Source: CAD feature listing. Evaluate the final solid. Frame: model axes, mm. A direction names the side the tool comes from. Coordinates: 2 decimals unless noted, no trailing zeros. Order: outer loops, then holes, each group sorted by start corner. A loop starts at its lowest first (then second) coordinate and runs counter-clockwise, first axis right, second up.
Item 1: Mould query, pull axis Y, two halves, no side actions, for faces 1 (the flat face through (12.98, 25.55, -54.55)), 2 (the cylindrical face through (15.63, 30.55, -67.76)), 3 (the flat face through (0, 10, -55)). Classes: released by +Y, released by -Y, zero draft, split by the parting line, or undercut.
Item 2: Section B-B on x = 1. Return the cut outline in (y, z).
Item 3: Section C-C on y = 25.5. Return the cut outline in (x, z).
Item 4: Section A-A on z = -2.62. Return the cut outline in (x, y).
Item 5: Ray query, line 1 (X direction, y = 6, z = -2.62); line 2 (Z direction, x = -5, y = 12); line 3 (X direction, y = 19, z = -33.5). Return the intervals inside material, ascending.
Item 6: Section D-D on z = -25. Return the cut outline in (x, y).
Item 7: Contact query for flat-ended pins moving along their axis: P1, Ø7, axis at y = 31, z = -61.5, coming from the -X side; P2, Ø1, axis at x = -3, z = -59.5, coming from the +Y side; P3, Ø8, axis at x = 0.5, z = -43.5, coming from the +Y side; P4, Ø8, axis at x = 2.5, z = -71, coming from the +Y side. Output: stop coordinate, or through.
Item 8: Reachability of faces 4 (the flat face through (13, 28, -50.07)), 5 (the flat face through (0, 29.5, -68)), 6 (the flat face through (0, 10, -6.622)), 7 (the flat face through (15.5, 12, -23)) from +Z, -Z, +X, -X, +Y, -Y: full face, straight path, thin tool, end or side. Return the list, or none.
from build123d import *

# Parameters (mm, degrees)
SKETCH1_W                  = 32
SKETCH1_H                  = 78.52
BOSS_EXTRUDE1_DEPTH        = 4
M3_CLEARANCE_HOLE1_D       = 3.6
M3_CLEARANCE_HOLE1_DEPTH   = 10
M3_CLEARANCE_HOLE1_TIP     = 1.081549114
BOSS_EXTRUDE2_DEPTH        = 17
BOSS_EXTRUDE3_DEPTH        = 17
SKETCH6_W                  = 32
SKETCH6_H                  = 1.5
SKETCH6_W_2                = 4
SKETCH6_H_2                = 6
BOSS_EXTRUDE4_DEPTH        = 8.5
SKETCH14_W                 = 4
SKETCH14_H                 = 18.45
BOSS_EXTRUDE5_DEPTH        = 6
FILLET1_R                  = 5
CHAMFER1_SIZE              = 3
CHAMFER2_SIZE              = 3
CUT_EXTRUDE1_DEPTH         = 87.102499383
CUT_EXTRUDE1_DEPTH_BACK    = 87.102499383
SKETCH15_W                 = 21
SKETCH15_H                 = 40.897809358
F_5_3_5_3_DIAMETER_HOLE1_D = 5.3
SKETCH19_W                 = 21
SKETCH19_H                 = 12
CUT_EXTRUDE2_DEPTH         = 10
CUT_EXTRUDE3_DEPTH         = 83.839546112
CUT_EXTRUDE3_DEPTH_BACK    = 83.839546112
SKETCH20_W                 = 6
SKETCH20_H                 = 2
CHAMFER3_SIZE              = 8.984147096
CHAMFER3_SIZE_2            = 4


with BuildPart() as part:
    # Sketch1 → Boss-Extrude1 (new body)
    with BuildSketch(Plane(origin=(0, 0, 0), x_dir=(1, 0, 0), z_dir=(0, 1, 0))):
        with Locations((0, 39.26)):
            Rectangle(SKETCH1_W, SKETCH1_H)
    extrude(amount=BOSS_EXTRUDE1_DEPTH)

    # M3 Clearance Hole1
    with Locations(Plane(origin=(0, 4, 0), x_dir=(1, 0, 0), z_dir=(0, 1, 0))):
        with Locations((-10, 73.52), (10, 73.52)):
            Hole(M3_CLEARANCE_HOLE1_D / 2, depth=M3_CLEARANCE_HOLE1_DEPTH)
            with Locations((0, 0, -(M3_CLEARANCE_HOLE1_DEPTH + M3_CLEARANCE_HOLE1_TIP / 2))):  # 118° drill point
                Cone(0, M3_CLEARANCE_HOLE1_D / 2, M3_CLEARANCE_HOLE1_TIP, mode=Mode.SUBTRACT)

    # Sketch5 → Boss-Extrude2 (add)
    with BuildSketch(Plane(origin=(0, 4, 0), x_dir=(1, 0, 0), z_dir=(0, 1, 0))):
        Polygon((16, 68.52), (-16, 68.52), (-16, 47.520000358), (-15.5, 47.520000358), (-10.5, 47.520000358), (10.5, 47.520000358), (15.5, 47.520000358), (16, 47.520000358), align=None)
    extrude(amount=BOSS_EXTRUDE2_DEPTH)

    # Sketch5<4> → Boss-Extrude3 (add)
    with BuildSketch(Plane(origin=(0, 4, 0), x_dir=(1, 0, 0), z_dir=(0, 1, 0))):
        Polygon((-10.5, 47.520000358), (-15.5, 47.520000358), (-15.5, 0), (15.5, 0), (15.5, 47.520000358), (10.5, 47.520000358), (10.5, 6.622191), (-10.5, 6.622191), align=None)
    extrude(amount=BOSS_EXTRUDE3_DEPTH)

    # Sketch6 → Boss-Extrude4 (add)
    with BuildSketch(Plane(origin=(0, 21, 0), x_dir=(1, 0, 0), z_dir=(0, 1, 0))):
        with Locations((0, 67.77)):
            Rectangle(SKETCH6_W, SKETCH6_H)
        with Locations((13.5, 53.07)):
            Rectangle(SKETCH6_W_2, SKETCH6_H_2)
        with Locations((-13.5, 53.07)):
            Rectangle(SKETCH6_W_2, SKETCH6_H_2)
    extrude(amount=BOSS_EXTRUDE4_DEPTH)

    # Sketch14 → Boss-Extrude5 (add)
    with BuildSketch(Plane(origin=(0, 29.5, 0), x_dir=(1, 0, 0), z_dir=(0, 1, 0))):
        with Locations((-13.5, 59.295)):
            Rectangle(SKETCH14_W, SKETCH14_H)
        with Locations((13.5, 59.295)):
            Rectangle(SKETCH14_W, SKETCH14_H)
    extrude(amount=BOSS_EXTRUDE5_DEPTH)

    # Fillet1
    # the kernel refuses this fillet: 5 mm, written as the material it adds along each edge
    with BuildSketch(Plane(origin=(-11.5, 29.5, -68.52), x_dir=(0, 1, 0), z_dir=(0, 0, 1)), Plane(origin=(11.5, 29.5, -68.52), x_dir=(-1, 0, 0), z_dir=(0, 0, 1))) as fillet1_piece_1:
        with BuildLine():
            CenterArc((FILLET1_R, -FILLET1_R), FILLET1_R, 90, 90)
            Line((0, -FILLET1_R), (0, 0))
            Line((0, 0), (FILLET1_R, 0))
        make_face()
    extrude(amount=1.5)
    with BuildSketch(Plane(origin=(-15.5, 29.5, -67.02), x_dir=(-1, 0, 0), z_dir=(0, 0, -1))) as fillet1_piece_2:
        with BuildLine():
            CenterArc((5, 2.179449472), FILLET1_R, 180, 25.841932763)
            Line((0, 2.179449472), (0, 0))
            Line((0, 0), (0.5, 0))
        make_face()
    extrude(amount=1.5)
    with BuildSketch(Plane(origin=(15.5, 29.5, -67.02), x_dir=(0, 1, 0), z_dir=(0, 0, -1))) as fillet1_piece_3:
        with BuildLine():
            CenterArc((2.179449472, 5), FILLET1_R, 244.158067237, 25.841932763)
            Line((0, 0.5), (0, 0))
            Line((0, 0), (2.179449472, 0))
        make_face()
    extrude(amount=1.5)

    # Chamfer1
    chamfer1_edges = [part.edges().sort_by_distance(p)[0] for p in [
        (-11.5, 29.5, -61.545),
        (11.5, 29.5, -61.545),
    ]]
    chamfer(chamfer1_edges, length=CHAMFER1_SIZE)

    # Chamfer2
    chamfer2_edges = [part.edges().sort_by_distance(p)[0] for p in [
        (11.5, 26.75, -56.07),
        (-11.5, 26.75, -56.07),
    ]]
    chamfer(chamfer2_edges, length=CHAMFER2_SIZE)

    # Sketch15 → Cut-Extrude1 (cut, two sides: drawn at the far end of the back side and taken through both)
    with BuildSketch(Plane(origin=(0, 4, 0), x_dir=(1, 0, 0), z_dir=(0, 1, 0)).offset(-CUT_EXTRUDE1_DEPTH_BACK)):
        with Locations((0, 27.071095679)):
            Rectangle(SKETCH15_W, SKETCH15_H)
    extrude(amount=CUT_EXTRUDE1_DEPTH + CUT_EXTRUDE1_DEPTH_BACK, mode=Mode.SUBTRACT)

    # Ø5.3 (5.3) Diameter Hole1 (through all)
    with Locations(Plane(origin=(0, 21, 0), x_dir=(1, 0, 0), z_dir=(0, 1, 0))):
        with Locations((-5, 52.220000358), (5, 52.220000358), (-5, 2.62), (5, 2.62)):
            Hole(F_5_3_5_3_DIAMETER_HOLE1_D / 2)

    # Sketch19 → Cut-Extrude2 (cut)
    with BuildSketch(Plane.XZ):
        with Locations((0, -53.520000358)):
            Rectangle(SKETCH19_W, SKETCH19_H)
    extrude(amount=-CUT_EXTRUDE2_DEPTH, mode=Mode.SUBTRACT)

    # Sketch20 → Cut-Extrude3 (cut, two sides: drawn at the far end of the back side and taken through both)
    with BuildSketch(Plane(origin=(0, 21, 0), x_dir=(1, 0, 0), z_dir=(0, 1, 0)).offset(-CUT_EXTRUDE3_DEPTH_BACK)):
        with Locations((0, 48.520000358)):
            Rectangle(SKETCH20_W, SKETCH20_H)
    extrude(amount=CUT_EXTRUDE3_DEPTH + CUT_EXTRUDE3_DEPTH_BACK, mode=Mode.SUBTRACT)

    # Chamfer3
    # the kernel refuses this chamfer: 8.984147096, 4 mm, written as the material it takes off along each edge
    with BuildSketch(Plane(origin=(-3, 10, -49.520000358), x_dir=(0, 0.9998768419809391, 0.015693975602887315), z_dir=(1, 0, 0))) as chamfer3_piece_1:
        Polygon((CHAMFER3_SIZE * 0.999876841938, -CHAMFER3_SIZE * 0.0156939756022), (-CHAMFER3_SIZE_2 * 0.0156939756029, -CHAMFER3_SIZE_2 * 0.999876841981), (0, 0), align=None)
    extrude(amount=6, mode=Mode.SUBTRACT)


solid = part.part
Answer list:
1. face 1: undercut
1. face 2: released by +Y
1. face 3: released by -Y
2. outline: (0, -78.52) - (4, -78.52) - (4, -68.52) - (29.5, -68.52) - (29.5, -67.02) - (21, -67.02) - (21, -49.52) - (18.98, -49.52) - (10, -53.52) - (10, -59.52) - (0, -59.52) - close; (0, -6.62) - (21, -6.62) - (21, 0) - (0, 0) - close
3. outline: (-16, -68.52) - (16, -68.52) - (16, -67.02) - (-16, -67.02) - close; (-15.5, -56.07) - (-14.5, -56.07) - (-11.5, -53.07) - (-11.5, -50.07) - (-15.5, -50.07) - close; (11.5, -53.07) - (14.5, -56.07) - (15.5, -56.07) - (15.5, -50.07) - (11.5, -50.07) - close
4. outline: (-16, 0) - (-7.65, 0) - (-7.65, 21) - (-15.5, 21) - (-15.5, 4) - (-16, 4) - close; (-2.35, 0) - (2.35, 0) - (2.35, 21) - (-2.35, 21) - close; (7.65, 0) - (16, 0) - (16, 4) - (15.5, 4) - (15.5, 21) - (7.65, 21) - close
5. line 1: x = -15.5 to -7.65, -2.35 to 2.35, 7.65 to 15.5
5. line 2: z = -68.52 to -54.87, -49.57 to -47.52, -6.62 to -5.27
5. line 3: x = -15.5 to -10.5, 10.5 to 15.5
6. outline: (-16, 0) - (-10.5, 0) - (-10.5, 21) - (-15.5, 21) - (-15.5, 4) - (-16, 4) - close; (10.5, 0) - (16, 0) - (16, 4) - (15.5, 4) - (15.5, 21) - (10.5, 21) - close
7. P1: stops at x = -15.5
7. P2: stops at y = 21
7. P3: passes through
7. P4: stops at y = 29.5
8. face 4: +Z, +X, -X, +Y
8. face 5: +Z, -Z, +Y
8. face 6: +Y, -Y
8. face 7: +Z, +X, +Y
